```python
from build123d import *

# Parameters (mm, degrees)
SALIENTE_EXTRUIR1_DEPTH = 100
CROQUIS2_R              = 6
CORTAR_EXTRUIR1_DEPTH   = 172.813852759


with BuildPart() as part:
    # Croquis1 → Saliente-Extruir1 (new body)
    with BuildSketch(Plane.XY):
        Polygon((-28, 125), (-28, -128), (28, -128), (28, 125), (25, 125), (25, -125), (-25, -125), (-25, 125), align=None)
    extrude(amount=SALIENTE_EXTRUIR1_DEPTH)

    # Croquis2 → Cortar-Extruir1 (cut, through all)
    with BuildSketch(Plane(origin=(28, 0, 0), x_dir=(0, 0, -1), z_dir=(1, 0, 0))):
        with Locations(Location((-81.704212475, 106.115669713, 0), (0, 0, 90))):
            Circle(CROQUIS2_R)
        with Locations(Location((-18.434102118, 106.115669713, 0), (0, 0, 90))):
            Circle(CROQUIS2_R)
        with Locations(Location((-18.434102118, 31.828375961, 0), (0, 0, 90))):
            Circle(CROQUIS2_R)
        with Locations(Location((-81.704212475, 31.828375961, 0), (0, 0, 90))):
            Circle(CROQUIS2_R)
    extrude(amount=-CORTAR_EXTRUIR1_DEPTH, mode=Mode.SUBTRACT)


solid = part.part
```
Can you work these out from the model? Positions are in its coordinate system, mm. A direction names the side the tool comes from. Round coordinates to 2 decimals unless told otherwise and drop trailing zeros. Loops run counter-clockwise (first coordinate to the right, second up) from the corner with the lowest first, then second, coordinate; pieces in that order, holes last.
Item 1: Will these pins go through, and if not, where does the flat tip stop? pin 1 Ø7 at (y, z) = (106.12, 81.7) entering from -X; pin 2 Ø15 at (x, z) = (-9, 27) entering from +Y.
Item 2: Suppose I cut it at B-B, the plane z = 32. Write out the boundary of the cut face in (x, y), then the cut area to 3 significant figures.
Item 3: Which directions (+Z, -Z, +X, -X, +Y, -Y) give clear straight access to the entire face, cutting with the end or side of a thin tool? Please do faces 1 (the flat face through (-25, -2, 49)), 2 (the cylindrical face through (26.521, 35.054, 86.763)).
Item 4: Suppose I cut it at A-A, the plane y = 51. Write out the boundary of the cut face in (x, z), then the cut area to 3 significant figures.
Item 5: Suppose I cut it at C-C, the plane x = -18.5. Write out the boundary of the cut face in (y, z), then the cut area to 3 significant figures.
Item 6: Please list where these lines run through material, in increasing order: L1, parallel to Y at x = -25.5, z = 19; L2, parallel to X at y = -4, z = 38; L3, parallel to Y at x = -24.5, z = 10.
Item 7: If we mould it in two halves opening along X, with no side actions, what happens to faces 3 (the flat face through (0, -125, 49)), 4 (the cylindrical face through (26.521, 35.054, 23.493)), 5 (the flat face through (-28, 0, 49)), 6 (the flat face through (25, 2, 49))? For each: +X half, -X half, draft (parallel to the pull), parting line (faces both ways), or undercut.
Reported:
1. pin 1: passes through
1. pin 2: stops at y = -125
2. outline: (-28, -128) - (28, -128) - (28, 125) - (25, 125) - (25, -125) - (-25, -125) - (-25, 125) - (-28, 125) - close
2. area: 1,670 mm2
3. face 1: +Z, -Z, +Y
3. face 2: +X, -X
4. outline: (-28, 0) - (-25, 0) - (-25, 100) - (-28, 100) - close; (25, 0) - (28, 0) - (28, 100) - (25, 100) - close
4. area: 600 mm2
5. outline: (-128, 0) - (-125, 0) - (-125, 100) - (-128, 100) - close
5. area: 300 mm2
6. L1: y = -128 to 25.86, 37.8 to 100.14, 112.09 to 125
6. L2: x = -28 to -25, 25 to 28
6. L3: y = -128 to -125
7. face 3: undercut
7. face 4: draft
7. face 5: -X half
7. face 6: undercut
